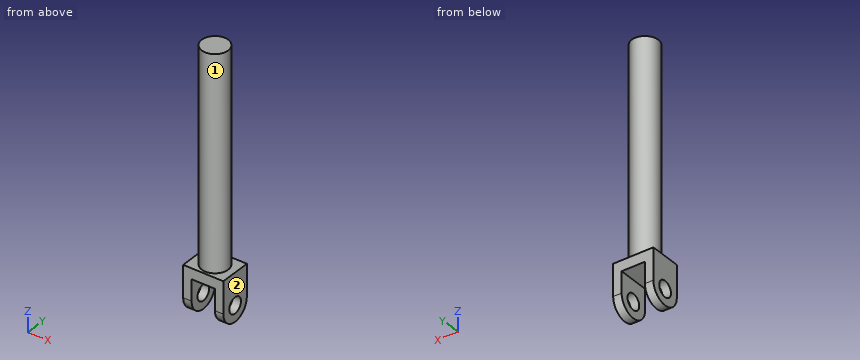
from build123d import *

# Parameters (mm, degrees)
SKETCH_1_R          = 7.5
EXTRUDE_1_DEPTH     = 19
SKETCH_2_W          = 22
SKETCH_2_H          = 35
CUT_EXTRUDE_1_DEPTH = 47.486557197
SKETCH_4_R          = 12.5
EXTRUDE_2_DEPTH     = 200


with BuildPart() as part:
    # 草图1 → 凸台-拉伸1 (new, symmetric)
    with BuildSketch(Plane(origin=(0, 0, 0), x_dir=(0, 0, -1), z_dir=(1, 0, 0))):
        with BuildLine():
            Line((0, -15), (-30, -15))
            Line((-30, -15), (-30, 15))
            Line((-30, 15), (0, 15))
            ThreePointArc((0, 15), (15, 0), (0, -15))
        make_face()
        Circle(SKETCH_1_R, mode=Mode.SUBTRACT)
    extrude(amount=EXTRUDE_1_DEPTH, both=True)

    # 草图2 → 切除-拉伸1 (cut, through all)
    with BuildSketch(Plane(origin=(0, 15, 0), x_dir=(1, 0, 0), z_dir=(0, 1, 0))):
        with Locations((0, -2.5)):
            Rectangle(SKETCH_2_W, SKETCH_2_H)
    extrude(amount=-CUT_EXTRUDE_1_DEPTH, mode=Mode.SUBTRACT)

    # 草图4 → 凸台-拉伸2 (add)
    with BuildSketch(Plane.XY.offset(30)):
        Circle(SKETCH_4_R)
    extrude(amount=EXTRUDE_2_DEPTH)


solid = part.part
Part model, mm, in its own coordinate system. Face numbers are marked on the shaded views. A direction names the side the tool comes from. Coordinates: 2 decimals unless noted, no trailing zeros. Order: outer loops, then holes, each group sorted by start corner. A loop starts at its lowest first (then second) coordinate and runs counter-clockwise, first axis right, second up.
(1) Pin check, flat tips, straight feed: pin 1 Ø5 at (y, z) = (11, 87) entering from -X; pin 2 Ø5 at (x, y) = (14.5, -3.5) entering from -Z; pin 3 Ø12 at (y, z) = (0.5, 39.5) entering from +X; pin 4 Ø12 at (y, z) = (0, 0) entering from -X. Stop position of each tip, or through.
Check sheet entries:
pin 1: stops at x = -9.17
pin 2: stops at z = -14.97
pin 3: stops at x = 12.5
pin 4: passes through
(2) Slice it at C-C, the plane z = 40.5. Write the cut outline in (x, y).
Check sheet entries:
outline: circle Ø25 at (0, 0)
(3) Slice it at B-B, the plane x = 0. Write the cut outline in (y, z).
Check sheet entries:
outline: (-15, 20) - (15, 20) - (15, 30) - (12.5, 30) - (12.5, 230) - (-12.5, 230) - (-12.5, 30) - (-15, 30) - close
(4) Probe L1, parallel to Z at x = 14.5, y = 0; L2, parallel to Y at x = 13.75, z = 0; L3, parallel to Z at x = 14, y = -13. List the from-to ranges inside material, lowest first.
Check sheet entries:
L1: z = -15 to -7.5, 7.5 to 30
L2: y = -15 to -7.5, 7.5 to 15
L3: z = -7.48 to 30
(5) Tool access for the marked faces 1 and 2: list every direction of +Z, -Z, +X, -X, +Y, -Y with a clear straight run to the whole face (end or side of a thin tool).
Check sheet entries:
face 1: +Z
face 2: +Z, -Z, +X, +Y, -Y
(6) Slice it at A-A, the plane y = 0. Write the cut outline in (x, z).
Check sheet entries:
outline: (-19, -15) - (-11, -15) - (-11, -7.5) - (-19, -7.5) - close; (-19, 7.5) - (-11, 7.5) - (-11, 20) - (11, 20) - (11, 7.5) - (19, 7.5) - (19, 30) - (12.5, 30) - (12.5, 230) - (-12.5, 230) - (-12.5, 30) - (-19, 30) - close; (11, -15) - (19, -15) - (19, -7.5) - (11, -7.5) - close
